For this review, use the dimensioned drawing (mm, ordinates from the lowest corner) and the shaded views. Round coordinates to 2 decimals unless told otherwise and drop trailing zeros. Loops run counter-clockwise (first coordinate to the right, second up) from the corner with the lowest first, then second, coordinate; pieces in that order, holes last. Notation, with made-up numbers: M -17.5,-11.75 L 24.5,-11.75 A18 cw 24.5,-0.75 Z; hole C -29,89.25 d4. An arc over 180 degrees is marked long. Use a Markdown table: item, result. Add a question column.
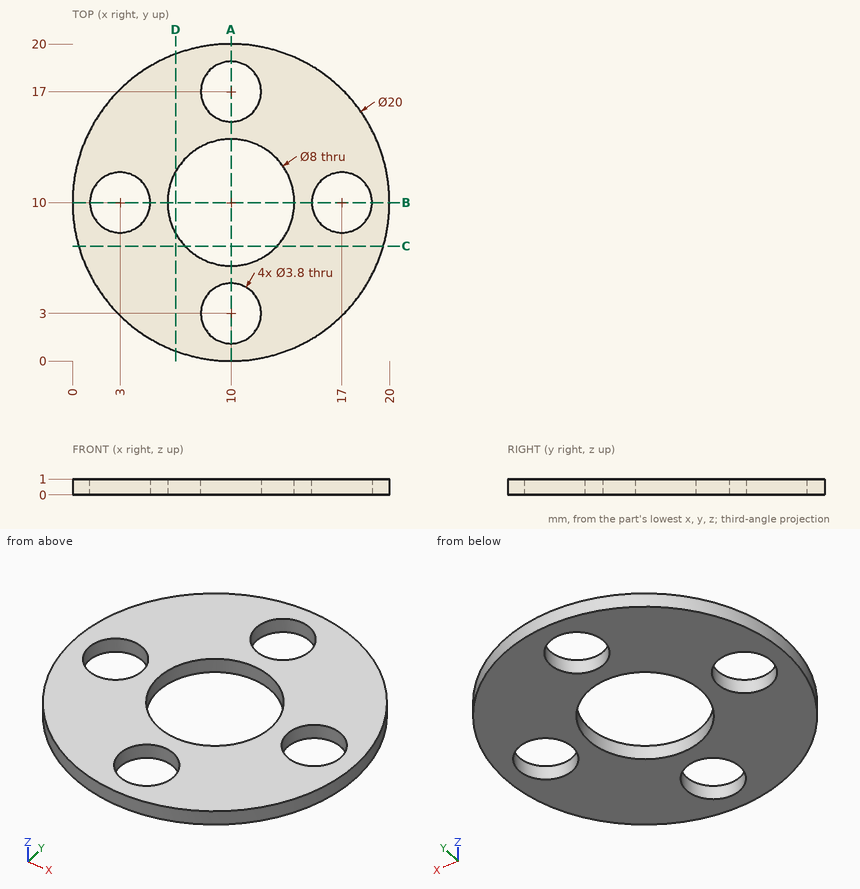
(1) Consider section D-D, the plane x = 6.5. Give the boundary of the cut face in (y, z), then the cut area to 3 significant figures.
(2) Consider section C-C, the plane y = 7.25. Give the boundary of the cut face in (x, z).
(3) Consider section A-A, the plane x = 10. Give the boundary of the cut face in (y, z).
(4) To check wall thickness, follow probe 1 along Y at (x, z) = (10, 0.8); probe 2 along X at (y, z) = (1.75, 0.9); probe 3 along X at (y, z) = (9.5, 0.5). State the ranges of each line that lie inside material, in increasing order.
Found:
| question | item | result |
|---|---|---|
| 1 | outline | M 0.63,0 L 8.06,0 L 8.06,1 L 0.63,1 Z; M 11.94,0 L 19.37,0 L 19.37,1 L 11.94,1 Z |
| 1 | area | 14.9 mm^2 |
| 2 | outline | M 0.39,0 L 7.1,0 L 7.1,1 L 0.39,1 Z; M 12.9,0 L 19.61,0 L 19.61,1 L 12.9,1 Z |
| 3 | outline | M 0,0 L 1.1,0 L 1.1,1 L 0,1 Z; M 4.9,0 L 6,0 L 6,1 L 4.9,1 Z; M 14,0 L 15.1,0 L 15.1,1 L 14,1 Z; M 18.9,0 L 20,0 L 20,1 L 18.9,1 Z |
| 4 | probe 1 | y = 0 to 1.1, 4.9 to 6, 14 to 15.1, 18.9 to 20 |
| 4 | probe 2 | x = 4.35 to 8.57, 11.43 to 15.65 |
| 4 | probe 3 | x = 0.01 to 1.17, 4.83 to 6.03, 13.97 to 15.17, 18.83 to 19.99 |
